Read the model definition and answer for the solid it produces. Units are mm, in the model's axes. Face numbers are marked on the shaded views. A direction names the side the tool comes from. Give positions to 0.01 mm unless a question says otherwise; leave off trailing zeros. Order: outer loops, then holes, each group sorted by start corner. A loop starts at its lowest first (then second) coordinate and runs counter-clockwise, first axis right, second up.
```python
from build123d import *

# Parameters (mm, degrees)
CUT_EXTRUDE1_DEPTH = 14
CIRPATTERN17_COUNT = 9
SKETCH6_R          = 1.5
CUT_EXTRUDE2_DEPTH = 10


with BuildPart() as part:
    # Sketch1 → Revolve1 (revolve)
    with BuildSketch(Plane(origin=(0, 0, 0), x_dir=(0, 0, -1), z_dir=(1, 0, 0)), mode=Mode.PRIVATE) as revolve1_sk:
        Polygon((0, 3), (0, 10), (14, 10), (14, 8), (19, 8), (19, 3), align=None)
    revolve(revolve1_sk.sketch.rotate(Axis((0, 0, 55), (0, 0, -1)), 90), axis=Axis((0, 0, 55), (0, 0, -1)))

    # Sketch2 → Cut-Extrude1 (cut)
    with BuildSketch(Plane.XY):
        with BuildLine():
            Line((3.674262438, 8.642141394), (3.75, 8.642141394))
            Line((3.75, 8.642141394), (3.75, 10.642141394))
            Line((3.75, 10.642141394), (-3.75, 10.642141394))
            Line((-3.75, 10.642141394), (-3.75, 8.642141394))
            Line((-3.75, 8.642141394), (-3.674262438, 8.642141394))
            ThreePointArc((-3.674262438, 8.642141394), (-3.199910012, 8.473080096), (-2.93940995, 8.04211413))
            ThreePointArc((-2.93940995, 8.04211413), (-2.331794227, 6.754484031), (-1.198957881, 5.892005073))
            Line((-1.198957881, 5.892005073), (1.198957881, 5.892005073))
            ThreePointArc((1.198957881, 5.892005073), (2.331794227, 6.754484031), (2.93940995, 8.04211413))
            ThreePointArc((2.93940995, 8.04211413), (3.199910012, 8.473080096), (3.674262438, 8.642141394))
        make_face()
    cut_extrude1 = extrude(amount=-CUT_EXTRUDE1_DEPTH, mode=Mode.SUBTRACT)

    # CirPattern17: Cut-Extrude1 ×9 about axis
    cirpattern17_axis = Axis((0, 0, 0), (0, 0, 1))
    for i in range(1, CIRPATTERN17_COUNT):
        add(cut_extrude1.rotate(cirpattern17_axis, i * 360 / CIRPATTERN17_COUNT), mode=Mode.SUBTRACT)

    # Sketch3 → Revolve2 (revolve)
    with BuildSketch(Plane(origin=(0, 0, 0), x_dir=(0, 0, -1), z_dir=(1, 0, 0)), mode=Mode.PRIVATE) as revolve2_sk:
        Polygon((0, 7.651144903), (0, 3.803703196), (1.5, 3.803703196), (1.5, 7.848623649), (0.856921938, 10.248623649), (-0.591966801, 9.860395082), align=None)
        Polygon((14.591966801, 9.860395082), (13.143078062, 10.248623649), (12.5, 7.848623649), (12.5, 3.803703196), (14, 3.803703196), (14, 7.651144903), align=None)
    revolve(revolve2_sk.sketch.rotate(Axis((0, 0, 55), (0, 0, -1)), 90), axis=Axis((0, 0, 55), (0, 0, -1)))

    # Sketch6 → Cut-Extrude2 (cut)
    with BuildSketch(Plane(origin=(0, 0, 0), x_dir=(1, 0, 0), z_dir=(0, 1, 0))):
        with Locations(Location((0, 16.759840403, 0), (0, 0, 270))):
            Circle(SKETCH6_R)
    extrude(amount=-CUT_EXTRUDE2_DEPTH, mode=Mode.SUBTRACT)


solid = part.part
```
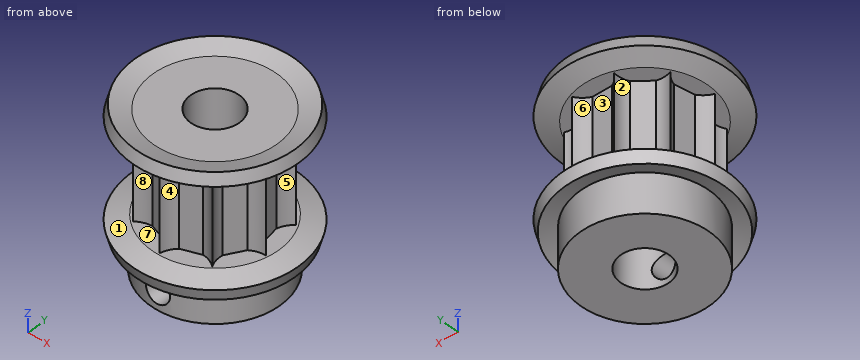
1) A tool of negligible diameter and unlimited length cuts with its end or side. For the marked faces 4, 5, 6, 7 and 8, from which of +Z, -Z, +X, -X, +Y, -Y can it reach the whole face along a straight path? Write none if from no direction.
Final values:
face 4: +X, -Y
face 5: +X
face 6: +Y
face 7: none
face 8: -Y
2) The part is cut by section C-C on z = -16.5. Determine the outline of the cut face in (x, y).
Final values:
outline: (-1.48, -7.86) - (-1.48, -2.61) arc R3 cw (long way) to (1.48, -2.61) - (1.48, -7.86) arc R8 ccw (long way) to start
3) Given pin 1 (2.5 mm diameter, centred on x = 0, z = -16.76, fed in from -Y); pin 2 (8 mm diameter, centred on x = 1, z = -4.5, fed in from +Y); pin 3 (2 mm diameter, centred on y = 2.5, z = -16, fed in from +X); pin 4 (4 mm diameter, centred on y = 0.5, z = -16, fed in from -X), each flat-ended and moving along its own axis, determine where each tip first touches the part or whether it passes through.
Final values:
pin 1: stops at y = 2.73
pin 2: stops at y = 10.25
pin 3: stops at x = 7.86
pin 4: stops at x = -10.01
4) The part is cut by section A-A on z = -9.75. Determine the outline of the cut face in (x, y), and give its area (3 significant figures).
Final values:
outline: (-7.49, -1.32) arc R3 cw to (-5.7, -1.91) - (-4.5, -3.98) arc R3 cw to (-4.89, -5.83) arc R3 cw to (-3.14, -5.13) - (-0.89, -5.95) arc R3 cw to (0, -7.61) arc R3 cw to (0.89, -5.95) - (3.14, -5.13) arc R3 cw to (4.89, -5.83) arc R3 cw to (4.5, -3.98) - (5.7, -1.91) arc R3 cw to (7.49, -1.32) arc R3 cw to (6.01, -0.16) - (5.59, 2.2) arc R3 cw to (6.59, 3.8) arc R3 cw to (4.71, 3.74) - (2.87, 5.28) arc R3 cw to (2.6, 7.15) arc R3 cw to (1.2, 5.89) - (-1.2, 5.89) arc R3 cw to (-2.6, 7.15) arc R3 cw to (-2.87, 5.28) - (-4.71, 3.74) arc R3 cw to (-6.59, 3.8) arc R3 cw to (-5.59, 2.2) - (-6.01, -0.16) arc R3 cw to start; hole circle Ø6 at (0, 0)
area: 92.7 mm2
5) The part is cut by section B-B on y = -5.5. Count the separate pieces of the cut face and the enclosed holes in it, and give its area (3 significant figures).
Final values:
separate pieces: 1
enclosed holes: 3
area: 155 mm2
6) Consider L1, parallel to Z at x = 0, y = -5.1; L2, parallel to Z at x = 3.75, y = -6.25; L3, parallel to Z at x = -0.25, y = 3.5. Determine where each line is inside the solid, lowest interval first.
Final values:
L1: z = -19 to -18.26, -15.26 to 0
L2: z = -19 to -12.5, -1.5 to 0
L3: z = -19 to 0
7) For a pull along Y with two mould halves and no side action, classify the marked faces 1, 2 and 3 as released by +Y, released by -Y, zero draft, split by the parting line, or undercut.
Final values:
face 1: split by the parting line
face 2: undercut
face 3: released by +Y
